from build123d import *

# Parameters (mm, degrees)
SKETCH1_W           = 50.8
SKETCH1_H           = 38.1
BOSS_EXTRUDE1_DEPTH = 50.292
BOSS_EXTRUDE2_DEPTH = 50.8
SKETCH3_R           = 12.1
CUT_EXTRUDE1_DEPTH  = 127
SKETCH4_W           = 57.912
SKETCH4_H           = 63.5
BOSS_EXTRUDE3_DEPTH = 5.08
SKETCH5_R           = 3.175
CUT_EXTRUDE2_DEPTH  = 5.08


with BuildPart() as part:
    # Sketch1 → Boss-Extrude1 (new body)
    with BuildSketch(Plane(origin=(0, 0, 0), x_dir=(1, 0, 0), z_dir=(0, 1, 0))):
        Rectangle(SKETCH1_W, SKETCH1_H)
    extrude(amount=BOSS_EXTRUDE1_DEPTH)

    # Sketch2 → Boss-Extrude2 (add)
    with BuildSketch(Plane(origin=(25.4, 0, 0), x_dir=(0, 0, -1), z_dir=(1, 0, 0))):
        with BuildLine():
            Line((-19.05, 0), (-14.119497191, -18.400886991))
            ThreePointArc((-14.119497191, -18.400886991), (0, -18.733351542), (14.119497191, -18.400886991))
            Line((14.119497191, -18.400886991), (19.05, 0))
            Line((19.05, 0), (-19.05, 0))
        make_face()
    extrude(amount=-BOSS_EXTRUDE2_DEPTH)

    # Sketch3 → Cut-Extrude1 (cut)
    with BuildSketch(Plane(origin=(25.4, 0, 0), x_dir=(0, 0, -1), z_dir=(1, 0, 0))):
        Circle(SKETCH3_R)
    extrude(amount=-CUT_EXTRUDE1_DEPTH, mode=Mode.SUBTRACT)

    # Sketch4 → Boss-Extrude3 (add)
    with BuildSketch(Plane(origin=(0, 50.292, 0), x_dir=(1, 0, 0), z_dir=(0, 1, 0))):
        Rectangle(SKETCH4_W, SKETCH4_H)
    extrude(amount=BOSS_EXTRUDE3_DEPTH)

    # Sketch5 → Cut-Extrude2 (cut)
    with BuildSketch(Plane(origin=(0, 55.372, 0), x_dir=(1, 0, 0), z_dir=(0, 1, 0))):
        with Locations((-22.606, 25.4)):
            Circle(SKETCH5_R)
        with Locations((-22.606, -25.4)):
            Circle(SKETCH5_R)
        with Locations((22.606, 25.4)):
            Circle(SKETCH5_R)
        with Locations((22.606, -25.4)):
            Circle(SKETCH5_R)
    extrude(amount=-CUT_EXTRUDE2_DEPTH, mode=Mode.SUBTRACT)


solid = part.part
CAD build for the part. Positions are in the model's coordinates, mm. A direction names the side the tool comes from. Round coordinates to 2 decimals unless told otherwise and drop trailing zeros. Loops run counter-clockwise (first coordinate to the right, second up) from the corner with the lowest first, then second, coordinate; pieces in that order, holes last.
(1) Cut at B-B (x = -15.5). Give the cut face in (y, z), plus the area to 3 significant figures.
(2) Cut at C-C (y = 4). Give the cut face in (x, z).
(3) Drop flat-ended pins along their axis: pin 1 (2 mm diameter, centred on y = -9.5, z = -8.5, fed in from -X); pin 2 (7.5 mm diameter, centred on x = 22.606, z = 25.4, fed in from +Y); pin 3 (15 mm diameter, centred on x = 4, y = 17.5, fed in from +Z); pin 4 (12 mm diameter, centred on x = -18.5, z = 17, fed in from -Y). Give the stop position or say it passes through.
(4) Two-plate mould, pull along Z, no slides. Class faces 1 (the flat face through (0, 55.372, 0)), 2 (the cylindrical face through (0.356, -18.733, 0.198)), 3 (the cylindrical face through (19.434, 52.868, 25.26)): +Z half, -Z half, draft (parallel to the pull), parting line (faces both ways), or undercut.
(5) Cut at A-A (z = -25.4). Give the cut face in (x, y).
(6) Wall check: line 1 along X through (y, z) = (53.8, -25.4); line 2 along Z through (x, y) = (-13, 46.5); line 3 along Y through (x, z) = (-21, 14). Give the ranges that are in metal, low to high.
(7) Which spindle directions (+Z, -Z, +X, -X, +Y, -Y) get a long thin tool onto all of the face, cutting with end or side? Do faces 4 (the flat face through (0, 25, -19.05)), 5 (the flat face through (25.4, 24, 0)), 6 (the flat face through (0, 25, 19.05)). Say none if no direction does.
(8) Cut at D-D (z = 0). Give the cut face in (x, y), plus the area to 3 significant figures.
Findings below:
1. outline: (-18.4, -14.12) - (0, -19.05) - (50.29, -19.05) - (50.29, -31.75) - (55.37, -31.75) - (55.37, 31.75) - (50.29, 31.75) - (50.29, 19.05) - (0, 19.05) - (-18.4, 14.12) arc R299.99 ccw to start; hole circle Ø24.2 at (0, 0)
1. area: 2,400 mm2
2. outline: (-25.4, -19.05) - (25.4, -19.05) - (25.4, -11.42) - (-25.4, -11.42) - close; (-25.4, 11.42) - (25.4, 11.42) - (25.4, 19.05) - (-25.4, 19.05) - close
3. pin 1: stops at x = -25.4
3. pin 2: stops at y = 55.37
3. pin 3: stops at z = 19.05
3. pin 4: stops at y = -18.53
4. face 1: draft
4. face 2: parting line
4. face 3: undercut
5. outline: (-28.96, 50.29) - (-25.78, 50.29) - (-25.78, 55.37) - (-28.96, 55.37) - close; (-19.43, 50.29) - (19.43, 50.29) - (19.43, 55.37) - (-19.43, 55.37) - close; (25.78, 50.29) - (28.96, 50.29) - (28.96, 55.37) - (25.78, 55.37) - close
6. line 1: x = -28.96 to -25.78, -19.43 to 19.43, 25.78 to 28.96
6. line 2: z = -19.05 to 19.05
6. line 3: y = -18.41 to 55.37
7. face 4: -Z, +X, -X, -Y
7. face 5: +Z, -Z, +X, -Y
7. face 6: +Z, +X, -X, -Y
8. outline: (-28.96, 50.29) - (-25.4, 50.29) - (-25.4, 12.1) - (25.4, 12.1) - (25.4, 50.29) - (28.96, 50.29) - (28.96, 55.37) - (-28.96, 55.37) - close; (-25.4, -18.73) - (25.4, -18.73) - (25.4, -12.1) - (-25.4, -12.1) - close
8. area: 2,570 mm2
